from build123d import *

# Parameters (mm, degrees)
SCHIZZO1_W                   = 42
SCHIZZO1_H                   = 46
SCHIZZO1_W_2                 = 34
SCHIZZO1_H_2                 = 38
ESTRUSIONE_SOTTILE1_DEPTH    = 30
SCHIZZO2_W                   = 42
SCHIZZO2_H                   = 46
ESTRUSIONE_ESTRUSIONE1_DEPTH = 4
SCHIZZO4_R                   = 1.5
TAGLIO_ESTRUSIONE1_DEPTH     = 4
RACCORDO1_R                  = 3
RACCORDO2_R                  = 3
RACCORDO3_R                  = 3
RACCORDO4_R                  = 3
ESTRUSIONE_ESTRUSIONE3_DEPTH = 5


with BuildPart() as part:
    # Schizzo1 → Estrusione-Sottile1 (new body)
    with BuildSketch(Plane.XY):
        Rectangle(SCHIZZO1_W, SCHIZZO1_H)
        Rectangle(SCHIZZO1_W_2, SCHIZZO1_H_2, mode=Mode.SUBTRACT)
    extrude(amount=ESTRUSIONE_SOTTILE1_DEPTH)

    # Schizzo2 → Estrusione-Estrusione1 (add)
    with BuildSketch(Plane.XY):
        Rectangle(SCHIZZO2_W, SCHIZZO2_H)
    extrude(amount=ESTRUSIONE_ESTRUSIONE1_DEPTH)

    # Schizzo4 → Taglio-Estrusione1 (cut)
    with BuildSketch(Plane.ZY.offset(21)):
        with Locations((22.540727145, 12.794949591)):
            Circle(SCHIZZO4_R)
        with Locations((22.540727145, 4.794949591)):
            Circle(SCHIZZO4_R)
        with Locations(Location((22.540727145, -4.794949591, 0), (0, 0, 180))):
            Circle(SCHIZZO4_R)
        with Locations(Location((22.540727145, -12.794949591, 0), (0, 0, 180))):
            Circle(SCHIZZO4_R)
    extrude(amount=-TAGLIO_ESTRUSIONE1_DEPTH, mode=Mode.SUBTRACT)

    # Raccordo1
    raccordo1_edges = [part.edges().sort_by_distance(p)[0] for p in [
        (-21, -23, 15),
    ]]
    fillet(raccordo1_edges, radius=RACCORDO1_R)

    # Raccordo2
    raccordo2_edges = [part.edges().sort_by_distance(p)[0] for p in [
        (21, -23, 15),
    ]]
    fillet(raccordo2_edges, radius=RACCORDO2_R)

    # Raccordo3
    raccordo3_edges = [part.edges().sort_by_distance(p)[0] for p in [
        (21, 23, 15),
    ]]
    fillet(raccordo3_edges, radius=RACCORDO3_R)

    # Raccordo4
    raccordo4_edges = [part.edges().sort_by_distance(p)[0] for p in [
        (-21, 23, 15),
    ]]
    fillet(raccordo4_edges, radius=RACCORDO4_R)

    # Schizzo3 → Estrusione-Estrusione3 (add)
    with BuildSketch(Plane.XY):
        with BuildLine():
            Line((-15.956647945, 23), (15.956647945, 23))
            add(Edge.make_bspline(
                [(15.956647945, 23), (8.114099812, 23.565784933), (9.021988807, 32.329235039), (5.183827034, 37.096841948), (3.979062469, 37.754360864)],
                knots=[0, 0, 0, 0, 0.676224636, 0.852915934, 0.852915934, 0.852915934, 0.852915934], degree=3))
            ThreePointArc((3.979062469, 37.754360864), (2.989638593, 37.736540073), (2.5, 36.876580054))
            Line((2.5, 36.876580054), (2.5, 32.299789094))
            ThreePointArc((2.5, 32.299789094), (0, 29.799789094), (-2.5, 32.299789094))
            Line((-2.5, 32.299789094), (-2.5, 36.876580054))
            ThreePointArc((-2.5, 36.876580054), (-2.989638593, 37.736540073), (-3.979062469, 37.754360864))
            add(Edge.make_bspline(
                [(-15.956647945, 23), (-8.114099812, 23.565784933), (-9.021988807, 32.329235039), (-5.183827034, 37.096841948), (-3.979062469, 37.754360864)],
                knots=[0, 0, 0, 0, 0.676224636, 0.852915934, 0.852915934, 0.852915934, 0.852915934], degree=3))
        make_face()
        with BuildLine():
            Line((2.5, -32.299789094), (2.5, -36.876580054))
            ThreePointArc((2.5, -36.876580054), (2.989638593, -37.736540073), (3.979062469, -37.754360864))
            add(Edge.make_bspline(
                [(15.956647945, -23), (8.114099812, -23.565784933), (9.021988807, -32.329235039), (5.183827034, -37.096841948), (3.979062469, -37.754360864)],
                knots=[0, 0, 0, 0, 0.676224636, 0.852915934, 0.852915934, 0.852915934, 0.852915934], degree=3))
            Line((15.956647945, -23), (-15.956647945, -23))
            add(Edge.make_bspline(
                [(-15.956647945, -23), (-8.114099812, -23.565784933), (-9.021988807, -32.329235039), (-5.183827034, -37.096841948), (-3.979062469, -37.754360864)],
                knots=[0, 0, 0, 0, 0.676224636, 0.852915934, 0.852915934, 0.852915934, 0.852915934], degree=3))
            ThreePointArc((-3.979062469, -37.754360864), (-2.989638593, -37.736540073), (-2.5, -36.876580054))
            Line((-2.5, -36.876580054), (-2.5, -32.299789094))
            ThreePointArc((-2.5, -32.299789094), (0, -29.799789094), (2.5, -32.299789094))
        make_face()
    extrude(amount=ESTRUSIONE_ESTRUSIONE3_DEPTH)


solid = part.part
For this review, take the finished solid that the model builds, in its own axes (mm). A direction names the side the tool comes from. Round coordinates to 2 decimals unless told otherwise and drop trailing zeros. Order: outer loops, then holes, each group sorted by start corner. A loop starts at its lowest first (then second) coordinate and runs counter-clockwise, first axis right, second up. Notation, with made-up numbers: (46, -40) -> (58, -40) arc R10 cw to (58, -34) -> close; hole circle Ø11 at (71, -36). An arc over 180 degrees is marked (long way). Put each result on its own line as item: value.
Q1. Machinability: for faces 1 (the cylindrical face through (-19.028, 12.22, 23.926)), 2 (the flat face through (0, 29, 5)), 3 (the flat face through (2.5, -35, 2)), 4 (the flat face through (0, 19, 17)), which of the approach directions +Z, -Z, +X, -X, +Y, -Y give a long, thin tool a straight path to every point of the face, cutting with its end or side? Answer none if there is none.
Check result:
face 1: -X
face 2: +Z, +X, -X, +Y
face 3: +Z, -Z, -Y
face 4: +Z
Q2. Mouldability with a two-part tool opening along X and no side actions: class faces 5 (the cylindrical face through (-19.03, 5.25, 23.97)), 6 (the cylindrical face through (-20.14, -22.1, 15.21)), 7 (the flat face through (0, -19, 17)), 8 (the cylindrical face through (-3.002, -37.744, 2.465)) as pulls with the +X half, pulls with the -X half, needs draft (parallel to the pull), parting line crosses it, or undercut.
Check result:
face 5: needs draft
face 6: pulls with the -X half
face 7: undercut
face 8: undercut
Q3. Add section B-B on x = 0. Write out the cut boundary in (y, z), plus the area to 3 significant figures.
Check result:
outline: (-29.8, 0) -> (29.8, 0) -> (29.8, 5) -> (23, 5) -> (23, 30) -> (19, 30) -> (19, 4) -> (-19, 4) -> (-19, 30) -> (-23, 30) -> (-23, 5) -> (-29.8, 5) -> close
area: 460 mm2
Q4. Insertion check: pin 1 Ø4.5 at (x, y) = (5.5, 28) entering from +Z; pin 2 Ø1 at (x, z) = (-9.5, 21.5) entering from -Y; pin 3 Ø1.4 at (y, z) = (34, 1.5) entering from -X. Each pin has a flat end and moves straight along its axis. Give the tip position at first contact, or say it passes through.
Check result:
pin 1: z = 5
pin 2: y = -23
pin 3: x = -7.26
Q5. Add section A-A on z = 15. Write out the cut boundary in (x, y).
Check result:
outline: (-21, -20) arc R3 ccw to (-18, -23) -> (18, -23) arc R3 ccw to (21, -20) -> (21, 20) arc R3 ccw to (18, 23) -> (-18, 23) arc R3 ccw to (-21, 20) -> close; hole (-17, -19) -> (17, -19) -> (17, 19) -> (-17, 19) -> close
Q6. Add section C-C on y = 2. Write out the cut boundary in (x, z), plus the area to 3 significant figures.
Check result:
outline: (-21, 0) -> (21, 0) -> (21, 30) -> (17, 30) -> (17, 4) -> (-17, 4) -> (-17, 30) -> (-21, 30) -> close
area: 376 mm2
Q7. For probe 1 along Y at (x, z) = (5.5, 14.5); probe 2 along X at (y, z) = (17.5, 7); probe 3 along Z at (x, y) = (-0.5, 6.5), list the stretches that pass through material, from the lowest coordinate up. Write a range as [from, to].
Check result:
probe 1: [-23, -19], [19, 23]
probe 2: [-21, -17], [17, 21]
probe 3: [0, 4]
